The listing builds one solid part. Answer for the finished solid, in the listing's coordinates (mm). A direction names the side the tool comes from. Give positions to 0.01 mm unless a question says otherwise; leave off trailing zeros. Write each loop counter-clockwise with the first axis right and the second up, starting at its lowest first coordinate (ties: lowest second). Pieces come first, ordered by that corner, then holes. Notation, with made-up numbers: (20.5, 82) -> (62.5, 82) arc R17 cw to (62.5, 102) -> close; hole circle Ø4 at (20, -30). An arc over 180 degrees is marked (long way). One line per question, with ' | ' between items.
from build123d import *

# Parameters (mm, degrees)
F0_R     = 1.875
F1_DEPTH = 1.5
F2_R     = 1


with BuildPart() as f1:
    # F0 (on Front) → F1 (new body)
    with BuildSketch(Plane.XZ):
        with BuildLine():
            Line((10.055, 0), (-10.055, 0))
            Line((-10.055, 0), (-10.055, -8))
            Line((-10.055, -8), (-8.09664, -9.664249))
            Line((-8.09664, -9.664249), (-8.09664, -15.664249))
            Line((-8.09664, -15.664249), (-10.055, -17.328498))
            Line((-10.055, -17.328498), (-10.055, -53.168498))
            Line((-10.055, -53.168498), (-6.7975, -58.630942))
            Line((-6.7975, -58.630942), (-3.54, -53.168498))
            Line((-3.54, -53.168498), (-3.54, -17.328498))
            ThreePointArc((-3.54, -17.328498), (0, -13.788498), (3.54, -17.328498))
            Line((3.54, -17.328498), (3.54, -53.168498))
            Line((3.54, -53.168498), (6.7975, -58.630942))
            Line((6.7975, -58.630942), (10.055, -53.168498))
            Line((10.055, -53.168498), (10.055, -17.328498))
            Line((10.055, -17.328498), (8.09664, -15.664249))
            Line((8.09664, -15.664249), (8.09664, -9.664249))
            Line((8.09664, -9.664249), (10.055, -8))
            Line((10.055, -8), (10.055, 0))
        make_face()
        with Locations((-6.739115, -2.67007)):
            Circle(F0_R, mode=Mode.SUBTRACT)
        with Locations((6.710854, -2.67007)):
            Circle(F0_R, mode=Mode.SUBTRACT)
    extrude(amount=F1_DEPTH)

    # F2
    f2_edges = [f1.edges().sort_by_distance(p)[0] for p in [
        (-8.09664, -0.75, -9.664249),
        (-8.09664, -0.75, -15.664249),
        (8.09664, -0.75, -9.664249),
        (8.09664, -0.75, -15.664249),
    ]]
    fillet(f2_edges, radius=F2_R)


solid = f1.part
Item 1: Find section A-A (z = -38.5). Write down the section's boundary in (x, y) (3 decimals), then the cut area to 3 significant figures.
Answers below:
outline: (-10.055, -1.5) -> (-3.54, -1.5) -> (-3.54, 0) -> (-10.055, 0) -> close; (3.54, -1.5) -> (10.055, -1.5) -> (10.055, 0) -> (3.54, 0) -> close | area: 19.5 mm²
Item 2: Determine the mould class of faces 1 (the face through (0, -1, 0)), 2 (the face through (-9.2, -0.7, -16.6)), 3 (the face through (8.4, -0.74, -55.94)), 4 (the face through (-10.055, -1, -4)) for opening direction Z: pulls with the +Z half, pulls with the -Z half, needs draft (parallel to the pull), parting line crosses it, or undercut.
Answers below:
face 1: pulls with the +Z half | face 2: undercut | face 3: pulls with the -Z half | face 4: needs draft
Item 3: Find section C-C (y = -0.5). Count the separate pieces of the cut face and the enclosed holes in it, then the cut area to 3 significant figures.
Answers below:
separate pieces: 1 | enclosed holes: 2 | area: 779 mm²
Item 4: Find section B-B (x = -6). Write down the section's boundary in (y, z), then the cut area to 3 significant figures.
Answers below:
outline: (-1.5, -57.29) -> (0, -57.29) -> (0, -4.39) -> (-1.5, -4.39) -> close; (-1.5, -0.95) -> (0, -0.95) -> (0, 0) -> (-1.5, 0) -> close | area: 80.8 mm²
Item 5: A tool of negligible diameter and unlimited length cuts with its end or side. For faces 5 (the face through (-5.192, -0.74, -55.938)), 6 (the face through (-8.45, -0.74, -55.86)), 7 (the face through (9.263, -0.74, -16.656)), 8 (the face through (-8.097, -1, -13)), from which of +Z, -Z, +X, -X, +Y, -Y can it reach the whole face along a straight path? Write none if from no direction.
Answers below:
face 5: -Z, +Y, -Y | face 6: -Z, -X, +Y, -Y | face 7: +X, +Y, -Y | face 8: -X, +Y, -Y
Item 6: Find section D-D (x = 0). Write down the section's boundary in (y, z).
Answers below:
outline: (-1.5, -13.79) -> (0, -13.79) -> (0, 0) -> (-1.5, 0) -> close
Item 7: Consider line 1 (X direction, y = -0.6, z = -41.5) (3 decimals); line 2 (X direction, y = -1.25, z = -3) (3 decimals); line 3 (Z direction, x = 8.75, y = -0.1). Determine where each line is inside the solid, lowest interval first. Write a range as [from, to].
Answers below:
line 1: [-10.055, -3.54], [3.54, 10.055] | line 2: [-10.055, -8.585], [-4.893, 4.865], [8.557, 10.055] | line 3: [-55.36, -16.22], [-9.11, 0]
